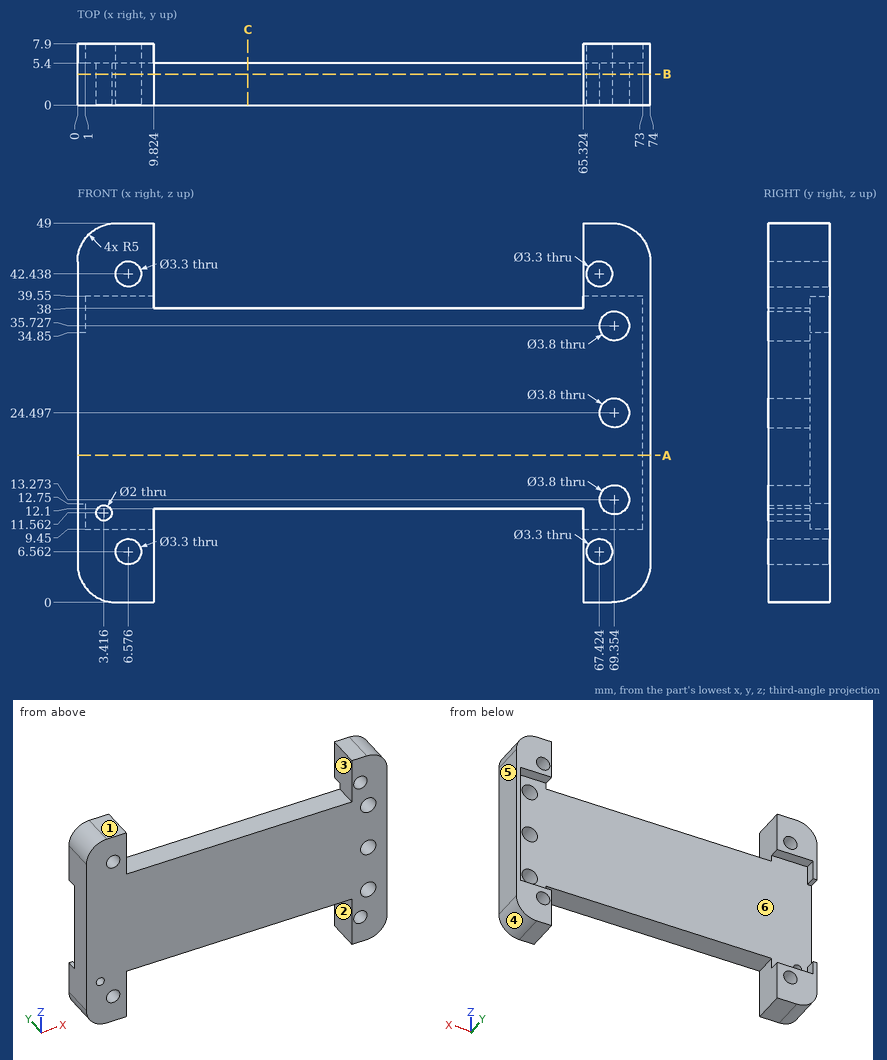
Design review of the part shown in the three views and the two pictorial views. Dimensions are in mm from the part's minimum x, y and z. A direction names the side the tool comes from. Round coordinates to 2 decimals unless told otherwise and drop trailing zeros. Write each loop counter-clockwise with the first axis right and the second up, starting at its lowest first coordinate (ties: lowest second). Pieces come first, ordered by that corner, then holes. Notation, with made-up numbers: (65.25, 18.25) - (80.25, 18.25) arc R10 ccw to (80.25, 27.25) - close; hole circle Ø5 at (47, -21.75). An arc over 180 degrees is marked (long way). Write item = value, one per line. Start each with the question number.
1. Draft analysis for pull direction Z (two halves, no side actions). For the marked faces 4, 5 and 6, state which applies: released by +Z, released by -Z, zero draft, split by the parting line, or undercut.
2. For pin 1 Ø3 at (x, y) = (3, 6) entering from -Z (1 decimal); pin 2 Ø1.6 at (x, y) = (39, 3) entering from -Z; pin 3 Ø2 at (x, y) = (36.5, 6.5) entering from +Z; pin 4 Ø6 at (x, z) = (61.5, 21) entering from +Y, all flat-tipped, find the tip position at first contact; note any pin that passes through.
3. For the marked faces 1, 2 and 3, list the 3-axis set-ups (+Z, -Z, +X, -X, +Y, -Y) from which the entire face can be reached by the end or side of a thin tool; tool diameter is ignored.
4. Wall thickness on L1, parallel to X at y = 4.5, z = 9 (1 decimal); L2, parallel to Z at x = 7, y = 7.75; L3, parallel to X at y = 2.75, z = 35.5: over which ranges is each line inside the solid? List them lowest first.
5. Consider section B-B on y = 4. Give the number of separate pieces and of enclosed holes in the cut face, plus the area to 3 significant figures.
6. Consider section A-A on z = 19. State the section outline as (x, y) points.
7. Consider section C-C on x = 22. State the section outline as (y, z) points, plus the area to 3 significant figures.
Evaluation:
q1.face_4 = released by -Z
q1.face_5 = zero draft
q1.face_6 = undercut
q2.pin_1 = 0
q2.pin_2 = 12.1
q2.pin_3 = through
q2.pin_4 = 5.4
q3.face_1 = +Z, +X, -X, +Y, -Y
q3.face_2 = -Z, +Y, -Y
q3.face_3 = +Z, +Y, -Y
q4.L1 = 0 to 9.8, 65.3 to 74
q4.L2 = 0 to 4.97, 8.16 to 9.45, 39.55 to 40.84, 44.03 to 49
q4.L3 = 0 to 67.47, 71.24 to 74
q5.separate_pieces = 1
q5.enclosed_holes = 8
q5.area = 2,250 mm2
q6.outline = (0, 0) - (74, 0) - (74, 7.9) - (73, 7.9) - (73, 5.4) - (0, 5.4) - close
q7.outline = (0, 12.1) - (5.4, 12.1) - (5.4, 38) - (0, 38) - close
q7.area = 140 mm2
